Study the drawing (mm; zero at the part's minimum x, y, z) and answer. Round coordinates to 2 decimals unless told otherwise and drop trailing zeros. Loops run counter-clockwise (first coordinate to the right, second up) from the corner with the lowest first, then second, coordinate; pieces in that order, holes last. Notation, with made-up numbers: (78.25, 20) -> (95.25, 20) arc R30 ccw to (95.25, 45) -> close; hole circle Ø3 at (66, -14.75). An arc over 180 degrees is marked (long way). Write each question's results on one line, items separated by ' | '. Start each with the question number.
(1) The part is cut by section A-A (z = 12.5). Determine the outline of the cut face in (x, y).
(2) The part is cut by section B-B (y = 10). Determine the outline of the cut face in (x, z), plus the area to 3 significant figures.
(3) A flat-ended cylindrical pin translates along its axis: pin 1 (8 mm diameter, centred on x = 15, z = 15, fed in from -Y). Find the tip coordinate at first contact, or state that the pin passes through.
(4) The part is cut by section C-C (z = 51). Determine the outline of the cut face in (x, y), plus the area to 3 significant figures.
(5) Determine the mould class of the marked faces 1, 2 and 3 for opening direction X: released by +X, released by -X, zero draft, split by the parting line, or undercut.
(6) The part is cut by section D-D (x = 20). Determine the outline of the cut face in (y, z), plus the area to 3 significant figures.
(7) Straight lines are drawn through the part: probe 1 along Z at (x, y) = (15, 8.25); probe 2 along X at (y, z) = (9.5, 51). For each, find the intervals that lie inside material, in ascending order.
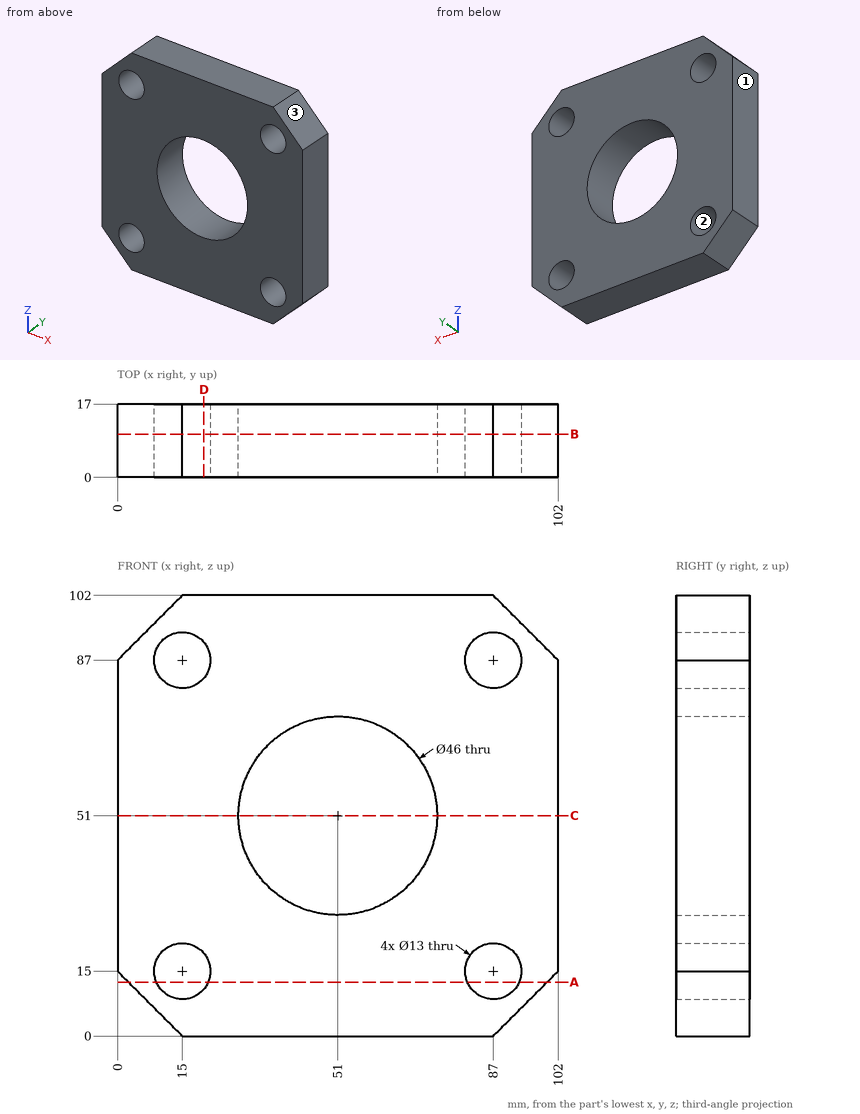
Checked values:
1) outline: (2.5, 0) -> (9, 0) -> (9, 17) -> (2.5, 17) -> close; (21, 0) -> (81, 0) -> (81, 17) -> (21, 17) -> close; (93, 0) -> (99.5, 0) -> (99.5, 17) -> (93, 17) -> close
2) outline: (0, 15) -> (15, 0) -> (87, 0) -> (102, 15) -> (102, 87) -> (87, 102) -> (15, 102) -> (0, 87) -> close; hole circle Ø13 at (15, 15); hole circle Ø13 at (15, 87); hole circle Ø46 at (51, 51); hole circle Ø13 at (87, 15); hole circle Ø13 at (87, 87) | area: 7,760 mm2
3) pin 1: passes through
4) outline: (0, 0) -> (28, 0) -> (28, 17) -> (0, 17) -> close; (74, 0) -> (102, 0) -> (102, 17) -> (74, 17) -> close | area: 952 mm2
5) face 1: released by -X | face 2: undercut | face 3: released by +X
6) outline: (0, 0) -> (17, 0) -> (17, 10.85) -> (0, 10.85) -> close; (0, 19.15) -> (17, 19.15) -> (17, 82.85) -> (0, 82.85) -> close; (0, 91.15) -> (17, 91.15) -> (17, 102) -> (0, 102) -> close | area: 1,450 mm2
7) probe 1: z = 0 to 8.5, 21.5 to 80.5, 93.5 to 102 | probe 2: x = 0 to 28, 74 to 102
